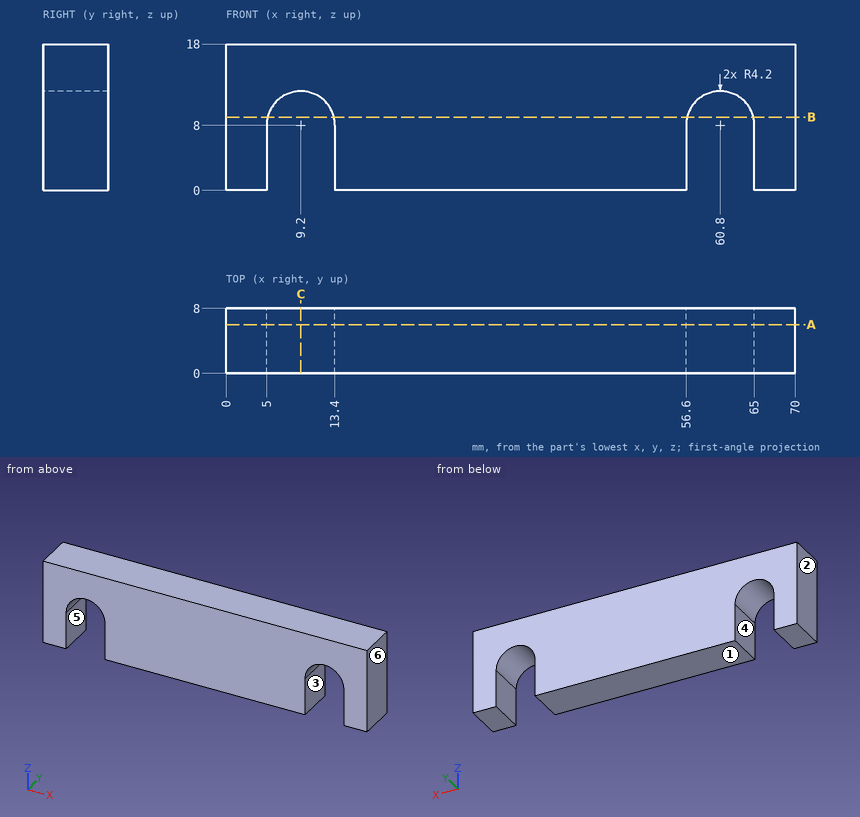
Answer from the drawing. Dimensions are ordinates in mm from the lowest x, y and z of the part. A direction names the side the tool comes from. Coordinates: 2 decimals unless noted, no trailing zeros. Loops run counter-clockwise (first coordinate to the right, second up) from the corner with the lowest first, then second, coordinate; pieces in that order, holes last. Notation, with made-up numbers: (-5, 59) -> (9, 59) arc R37 ccw to (9, 97) -> close; hole circle Ø10 at (-1.75, 22.5). An arc over 180 degrees is marked (long way). Answer in a Markdown table with one row per item.
Item 1: For a pull along X with two mould halves and no side action, classify the marked faces 1, 2, 3 and 4 as released by +X, released by -X, zero draft, split by the parting line, or undercut.
Returned:
| item | result |
|---|---|
| face 1 | zero draft |
| face 2 | released by -X |
| face 3 | undercut |
| face 4 | undercut |
Item 2: Straight lines are drawn through the part: line 1 along X through (y, z) = (6, 4.5); line 2 along X through (y, z) = (3.5, 11.25); line 3 along Z through (x, y) = (8, 3). For each, find the intervals that lie inside material, in ascending order. Write a range as [from, to].
Returned:
| item | result |
|---|---|
| line 1 | x = [0, 5], [13.4, 56.6], [65, 70] |
| line 2 | x = [0, 6.54], [11.86, 58.14], [63.46, 70] |
| line 3 | z = [12.02, 18] |
Item 3: A cutting plane is placed at C-C on x = 9.2. Determine the outline of the cut face in (y, z), plus the area to 3 significant figures.
Returned:
| item | result |
|---|---|
| outline | (0, 12.2) -> (8, 12.2) -> (8, 18) -> (0, 18) -> close |
| area | 46.4 mm^2 |
Item 4: A cutting plane is placed at A-A on y = 6. Determine the outline of the cut face in (x, z).
Returned:
| item | result |
|---|---|
| outline | (0, 0) -> (5, 0) -> (5, 8) arc R4.2 cw to (13.4, 8) -> (13.4, 0) -> (56.6, 0) -> (56.6, 8) arc R4.2 cw to (65, 8) -> (65, 0) -> (70, 0) -> (70, 18) -> (0, 18) -> close |
Item 5: For the marked faces 5 and 6, determine the directions among +Z, -Z, +X, -X, +Y, -Y from which every point of the face is accessible in a straight line to the end or side of a thin tool.
Returned:
| item | result |
|---|---|
| face 5 | -Z, +Y, -Y |
| face 6 | +Z, -Z, +X, +Y, -Y |
Item 6: A cutting plane is placed at B-B on z = 9. Determine the outline of the cut face in (x, y), plus the area to 3 significant figures.
Returned:
| item | result |
|---|---|
| outline | (0, 0) -> (5.12, 0) -> (5.12, 8) -> (0, 8) -> close; (13.28, 0) -> (56.72, 0) -> (56.72, 8) -> (13.28, 8) -> close; (64.88, 0) -> (70, 0) -> (70, 8) -> (64.88, 8) -> close |
| area | 429 mm^2 |
